Work out the finished part from the listing and answer in its coordinate system (mm). A direction names the side the tool comes from. Round coordinates to 2 decimals unless told otherwise and drop trailing zeros. Order: outer loops, then holes, each group sorted by start corner. A loop starts at its lowest first (then second) coordinate and runs counter-clockwise, first axis right, second up. Notation, with made-up numbers: (27.5, 40) - (78.5, 40) arc R13 cw to (78.5, 46) - close; hole circle Ø8 at (44, 40). An arc over 180 degrees is marked (long way). Put each result on its own line as item: value.
```python
from build123d import *

# Parameters (mm, degrees)
SKETCH_1_R             = 8
EXTRUDE_1_DEPTH        = 150
SKETCH_5_W             = 1
SKETCH_5_H             = 1.2
PATTERN_LINEAR_1_COUNT = 2
PATTERN_LINEAR_1_PITCH = 74


with BuildPart() as part:
    # 草图1 → 凸台-拉伸1 (new, symmetric)
    with BuildSketch(Plane(origin=(0, 0, 0), x_dir=(1, 0, 0), z_dir=(0, 1, 0))):
        with Locations(Location((0, 0, 0), (0, 0, 270))):
            Circle(SKETCH_1_R)
    extrude(amount=EXTRUDE_1_DEPTH, both=True)

    # 草图3 → M5 螺纹孔1 (revolve, cut)
    with BuildSketch(Plane(origin=(0, 150, 0), x_dir=(0, 0, 1), z_dir=(1, 0, 0))):
        Polygon((0, 0), (0, 15.2618073), (2.1, 14), (2.1, 0), align=None)
    hole_wizard_m5_1 = revolve(axis=Axis((0, 156.35, 0), (0, -1, 0)), mode=Mode.SUBTRACT)

    # 镜向1: M5 螺纹孔1 across plane
    add(hole_wizard_m5_1.mirror(Plane.ZX), mode=Mode.SUBTRACT)

    # 草图5 → 切除-旋转1 (revolve, cut)
    with BuildSketch(Plane.XY, mode=Mode.PRIVATE) as cut_revolve_1_sk:
        with Locations((7.5, -110.6)):
            Rectangle(SKETCH_5_W, SKETCH_5_H)
    cut_revolve_1 = revolve(cut_revolve_1_sk.sketch.rotate(Axis((0, 150, 0), (0, -1, 0)), 90), axis=Axis((0, 150, 0), (0, -1, 0)), mode=Mode.SUBTRACT)

    # 阵列(线性)1: 切除-旋转1 ×2
    with Locations(*[(0, i * PATTERN_LINEAR_1_PITCH, 0) for i in range(1, PATTERN_LINEAR_1_COUNT)]):
        add(cut_revolve_1, mode=Mode.SUBTRACT)


solid = part.part
```
1) Straight lines are drawn through the part: L1, parallel to Y at x = -6.5, z = 3.5; L2, parallel to Z at x = 0, y = 146.25. For each, find the intervals that lie inside material, in ascending order. Write a range as from..to.
Findings below:
L1: y = -150..-111.2, -110..-37.2, -36..150
L2: z = -8..-2.1, 2.1..8
2) For a pull along Y with two mould halves and no side action, classify faces 1 (the cylindrical face through (6.21, -110.59, 3.23)), 2 (the cylindrical face through (-7.81, 58.3, -1.73)), 3 (the flat face through (6, -111.2, -4)), 4 (the flat face through (-2, 150, 2)) as pulls with the +Y half, pulls with the -Y half, needs draft (parallel to the pull), parting line crosses it, or undercut.
Findings below:
face 1: undercut
face 2: needs draft
face 3: undercut
face 4: pulls with the +Y half
3) For faces 5 (the flat face through (6, -37.2, -4)), 6 (the flat face through (-2, -150, 2)), determine the directions among +Z, -Z, +X, -X, +Y, -Y from which every point of the face is accessible in a straight line to the end or side of a thin tool.
Findings below:
face 5: none
face 6: +Z, -Z, +X, -X, -Y
4) A cutting plane is placed at A-A on y = 64. Write down the section's boundary in (x, z).
Findings below:
outline: circle Ø16 at (0, 0)
5) Given pin 1 Ø3 at (y, z) = (-91.5, 1) entering from -X; pin 2 Ø2.5 at (x, z) = (0, 0) entering from +Y; pin 3 Ø5 at (x, y) = (3, -88) entering from -Z, each flat-ended and moving along its own axis, determine where each tip first touches the part or whether it passes through.
Findings below:
pin 1: stops at x = -8
pin 2: stops at y = 135.49
pin 3: stops at z = -7.98
